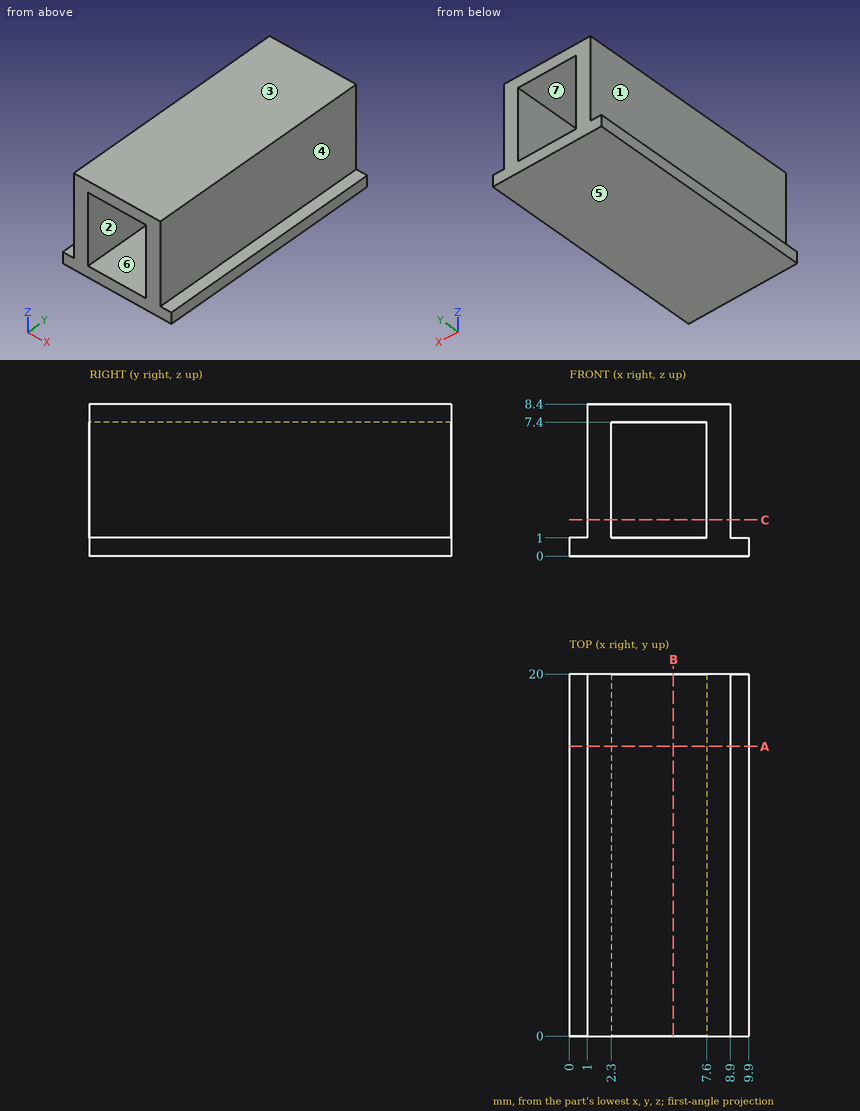
Geometry check sheet. Reference: drawing and pictorial views, mm from the part's lowest x, y, z. A direction names the side the tool comes from. Coordinates: 2 decimals unless noted, no trailing zeros. Order: outer loops, then holes, each group sorted by start corner. A loop starts at its lowest first (then second) coordinate and runs counter-clockwise, first axis right, second up.
1. Sectioned sample at B-B, the plane x = 5.75. Record the cut outline in (y, z), and give its area (3 significant figures).
Results found:
outline: (0, 0) - (20, 0) - (20, 1) - (0, 1) - close; (0, 7.4) - (20, 7.4) - (20, 8.4) - (0, 8.4) - close
area: 40.0 mm2
2. Scan lines: line 1 (Z direction, x = 3.75, y = 9.75); line 2 (X direction, y = 15.5, z = 2.75); line 3 (X direction, y = 7.25, z = 8.25). Record each from-to range of solid material in increasing order.
Results found:
line 1: z = 0 to 1, 7.4 to 8.4
line 2: x = 1 to 2.3, 7.6 to 8.9
line 3: x = 1 to 8.9
3. Go/stop test with flat-tipped pins: pin 1 Ø3 at (x, y) = (8, 17) entering from -Z; pin 2 Ø2 at (y, z) = (5, 4) entering from +X; pin 3 Ø5 at (y, z) = (14.5, 4) entering from -X; pin 4 Ø1.5 at (x, z) = (6, 4) entering from -Y. Record where each tip stops, or that it passes through.
Results found:
pin 1: stops at z = 0
pin 2: stops at x = 8.9
pin 3: stops at x = 1
pin 4: passes through
4. Release check for a two-part mould opening along X. For the marked faces 4, 5, 6 and 7 record: +X half, -X half, draft (parallel to the pull), parting line (faces both ways), or undercut.
Results found:
face 4: +X half
face 5: draft
face 6: undercut
face 7: undercut
5. Sectioned sample at C-C, the plane z = 2. Record the cut outline in (x, y).
Results found:
outline: (1, 0) - (2.3, 0) - (2.3, 20) - (1, 20) - close; (7.6, 0) - (8.9, 0) - (8.9, 20) - (7.6, 20) - close
6. Set-up check for the marked faces 1, 2 and 3: record each of +Z, -Z, +X, -X, +Y, -Y from which the full face is reachable in a straight line by a thin tool's end or side.
Results found:
face 1: +Z, -X, +Y, -Y
face 2: +Y, -Y
face 3: +Z, +X, -X, +Y, -Y
7. Sectioned sample at A-A, the plane y = 16. Record the cut outline in (x, z).
Results found:
outline: (0, 0) - (9.9, 0) - (9.9, 1) - (8.9, 1) - (8.9, 8.4) - (1, 8.4) - (1, 1) - (0, 1) - close; hole (2.3, 1) - (7.6, 1) - (7.6, 7.4) - (2.3, 7.4) - close
